from build123d import *

# Parameters (mm, degrees)
SKETCH1_W           = 37
SKETCH1_H           = 35
SKETCH1_W_2         = 23
SKETCH1_H_2         = 13
BOSS_EXTRUDE1_DEPTH = 3
FILLET1_R           = 2


with BuildPart() as part:
    # Sketch1 → Boss-Extrude1 (new body)
    with BuildSketch(Plane(origin=(0, 0, 0), x_dir=(1, 0, 0), z_dir=(0, 1, 0))):
        Rectangle(SKETCH1_W, SKETCH1_H)
        with Locations((0, 9)):
            Rectangle(SKETCH1_W_2, SKETCH1_H_2, mode=Mode.SUBTRACT)
        with BuildLine():
            Line((-13, -10.5), (13, -10.5))
            ThreePointArc((13, -10.5), (15, -12.5), (13, -14.5))
            Line((13, -14.5), (-13, -14.5))
            ThreePointArc((-13, -14.5), (-15, -12.5), (-13, -10.5))
        make_face(mode=Mode.SUBTRACT)
    extrude(amount=BOSS_EXTRUDE1_DEPTH)

    # Fillet1
    fillet1_edges = [part.edges().sort_by_distance(p)[0] for p in [
        (18.5, 1.5, 17.5),
        (-18.5, 1.5, 17.5),
        (-18.5, 1.5, -17.5),
        (18.5, 1.5, -17.5),
    ]]
    fillet(fillet1_edges, radius=FILLET1_R)


solid = part.part
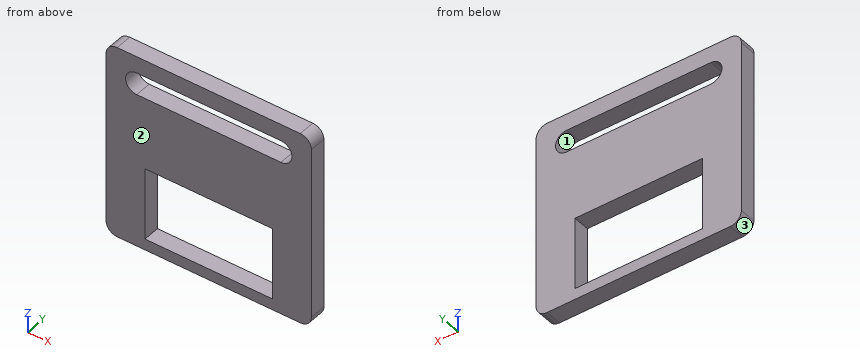
For this review, take the finished solid that the model builds, in its own axes (mm). Face numbers are marked on the shaded views. Give positions to 0.01 mm unless a question says otherwise; leave off trailing zeros. Loops run counter-clockwise (first coordinate to the right, second up) from the corner with the lowest first, then second, coordinate; pieces in that order, holes last. Notation, with made-up numbers: M 25,76 L 32,76 A25 cw 32,106 Z; hole C -3.75,-38 d7. An arc over 180 degrees is marked long. Answer as a JSON object with one key per item and string values. Group by question number.
Q1. Add section A-A on z = 12.5. Give the boundary of the cut face in (x, y), and give its area (3 significant figures).
Q2. Add section C-C on y = 1.4. Give the boundary of the cut face in (x, z).
Q3. Mouldability with a two-part tool opening along X and no side actions: class the marked faces 1, 2 and 3 as +X half, -X half, draft (parallel to the pull), parting line (faces both ways), or undercut.
Q4. For probe 1 along Z at (x, y) = (7, 2.85); probe 2 along X at (y, z) = (1.9, -6); probe 3 along Z at (x, y) = (12, 1.95), list the stretches that pass through material, from the lowest coordinate up. Write a range as [from, to].
Q5. Add section B-B on x = 3.5. Give the boundary of the cut face in (y, z).
Q6. Insertion check: P1, Ø1.5, axis at x = -4.5, z = 12.5, coming from the -Y side. The pin has a flat end and moves straight along its axis. Give the tip position at first contact, or say it passes through.
Checked values:
{
 "1": {"outline": "M -18.5,0 L -15,0 L -15,3 L -18.5,3 Z; M 15,0 L 18.5,0 L 18.5,3 L 15,3 Z", "area": "21.0 mm²"},
 "2": {"outline": "M -18.5,-15.5 A2 ccw -16.5,-17.5 L 16.5,-17.5 A2 ccw 18.5,-15.5 L 18.5,15.5 A2 ccw 16.5,17.5 L -16.5,17.5 A2 ccw -18.5,15.5 Z; hole M -13,10.5 L 13,10.5 A2 ccw 13,14.5 L -13,14.5 A2 ccw Z; hole M -11.5,-15.5 L 11.5,-15.5 L 11.5,-2.5 L -11.5,-2.5 Z"},
 "3": {"face 1": "undercut", "face 2": "draft", "face 3": "-X half"},
 "4": {"probe 1": "[-17.5, -15.5], [-2.5, 10.5], [14.5, 17.5]", "probe 2": "[-18.5, -11.5], [11.5, 18.5]", "probe 3": "[-17.5, 10.5], [14.5, 17.5]"},
 "5": {"outline": "M 0,-17.5 L 3,-17.5 L 3,-15.5 L 0,-15.5 Z; M 0,-2.5 L 3,-2.5 L 3,10.5 L 0,10.5 Z; M 0,14.5 L 3,14.5 L 3,17.5 L 0,17.5 Z"},
 "6": {"P1": "through"}
}
